Verification items for this drawing (mm, ordinates from the low corner). A direction names the side the tool comes from. Round coordinates to 2 decimals unless told otherwise and drop trailing zeros. Loops run counter-clockwise (first coordinate to the right, second up) from the corner with the lowest first, then second, coordinate; pieces in that order, holes last. Notation, with made-up numbers: (-2, 82) -> (44, 82) arc R17 ccw to (44, 88) -> close; hole circle Ø9 at (28.5, -3.5). An arc over 180 degrees is marked (long way). Use a Markdown table: item, result. Add a question column.
Q1. Gauge pin test, flat ends, axial feed: P1, Ø1, axis at y = 1.5, z = 8, coming from the -X side; P2, Ø2, axis at y = 5.5, z = 18, coming from the +X side; P3, Ø1, axis at y = 3.5, z = 27.5, coming from the -X side. Record the tip position at first contact, or that the pin passes through.
Q2. Material ranges on L1, parallel to X at y = 7.3, z = 16; L2, parallel to X at y = 7.75, z = 14.5; L3, parallel to Y at x = 8.5, z = 17.5, recorded low to high.
Q3. Sectioned sample at A-A, the plane x = 16. Enter the section's corners in (y, z).
Q4. Release check for a two-part mould opening along X. For the marked faces 3, 4 and 5 record: released by +X, released by -X, zero draft, split by the parting line, or undercut.
Q5. Sectioned sample at D-D, the plane z = 6. Enter the section's corners in (x, y), then the cut area to 3 significant figures.
Q6. Set-up check for the marked faces 1 and 2: record each of +Z, -Z, +X, -X, +Y, -Y from which the full face is reachable in a straight line by a thin tool's end or side.
Q7. Sectioned sample at B-B, the plane y = 3. Enter the section's corners in (x, z), then the cut area to 3 significant figures.
Q8. Sectioned sample at C-C, the plane x = 3. Enter the section's corners in (y, z).
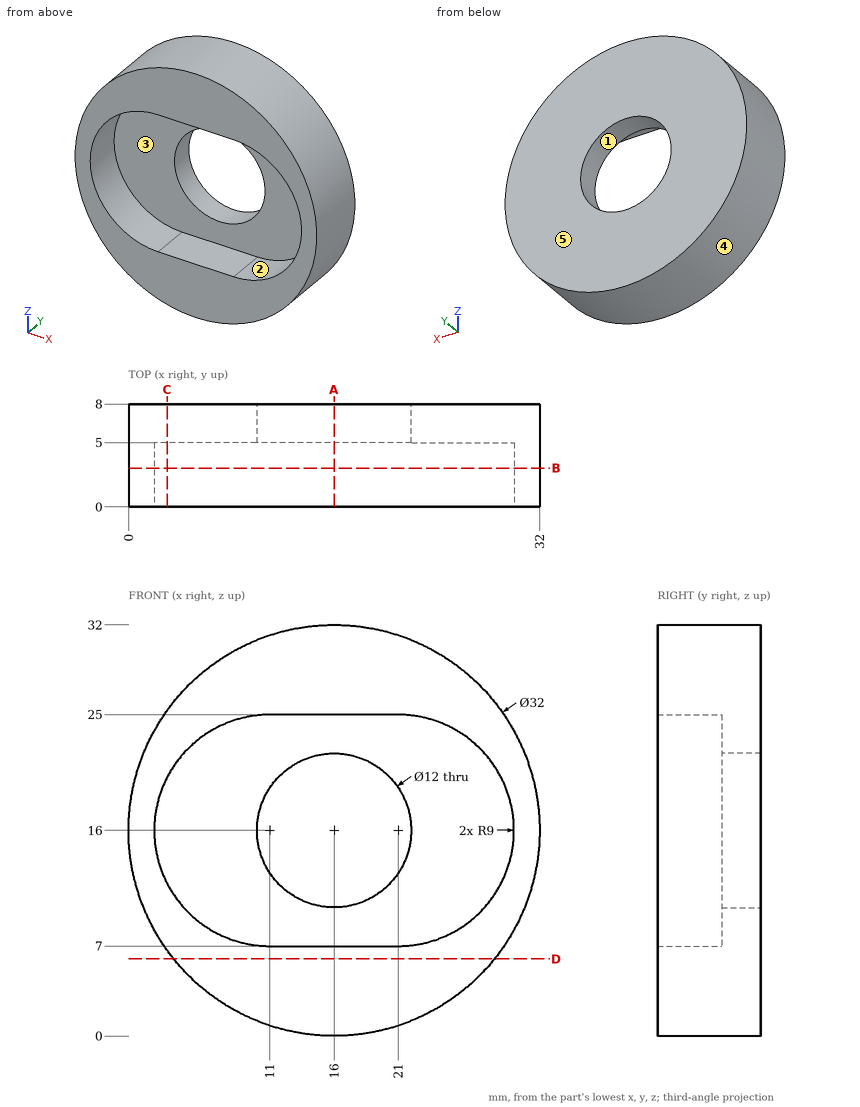
Values:
| question | item | result |
|---|---|---|
| 1 | P1 | x = 1.87 |
| 1 | P2 | x = 31.97 |
| 1 | P3 | x = 4.38 |
| 2 | L1 | 0 to 10, 22 to 32 |
| 2 | L2 | 0.07 to 10.19, 21.81 to 31.93 |
| 2 | L3 | 5 to 8 |
| 3 | outline | (0, 0) -> (8, 0) -> (8, 10) -> (5, 10) -> (5, 7) -> (0, 7) -> close; (0, 25) -> (5, 25) -> (5, 22) -> (8, 22) -> (8, 32) -> (0, 32) -> close |
| 4 | face 3 | undercut |
| 4 | face 4 | split by the parting line |
| 4 | face 5 | zero draft |
| 5 | outline | (3.51, 0) -> (28.49, 0) -> (28.49, 8) -> (3.51, 8) -> close |
| 5 | area | 200 mm^2 |
| 6 | face 1 | +Y, -Y |
| 6 | face 2 | -Y |
| 7 | outline | circle Ø32 at (16, 16); hole (11, 7) -> (21, 7) arc R9 ccw to (21, 25) -> (11, 25) arc R9 ccw to start |
| 7 | area | 370 mm^2 |
| 8 | outline | (0, 6.67) -> (8, 6.67) -> (8, 25.33) -> (0, 25.33) -> (0, 20.12) -> (5, 20.12) -> (5, 11.88) -> (0, 11.88) -> close |
